The figure shows three views and two pictorial views of one solid part (mm, origin at its lowest corner). Answer the questions. A direction names the side the tool comes from. Give positions to 0.01 mm unless a question says otherwise; leave off trailing zeros. Order: outer loops, then holes, each group sorted by start corner. A loop starts at its lowest first (then second) coordinate and runs counter-clockwise, first axis right, second up. Notation, with made-up numbers: (30, 12.5) - (58, 12.5) arc R9 cw to (58, 26.5) - close; hole circle Ø7 at (84, -27). An arc over 180 degrees is marked (long way). Write item = value, one per line.
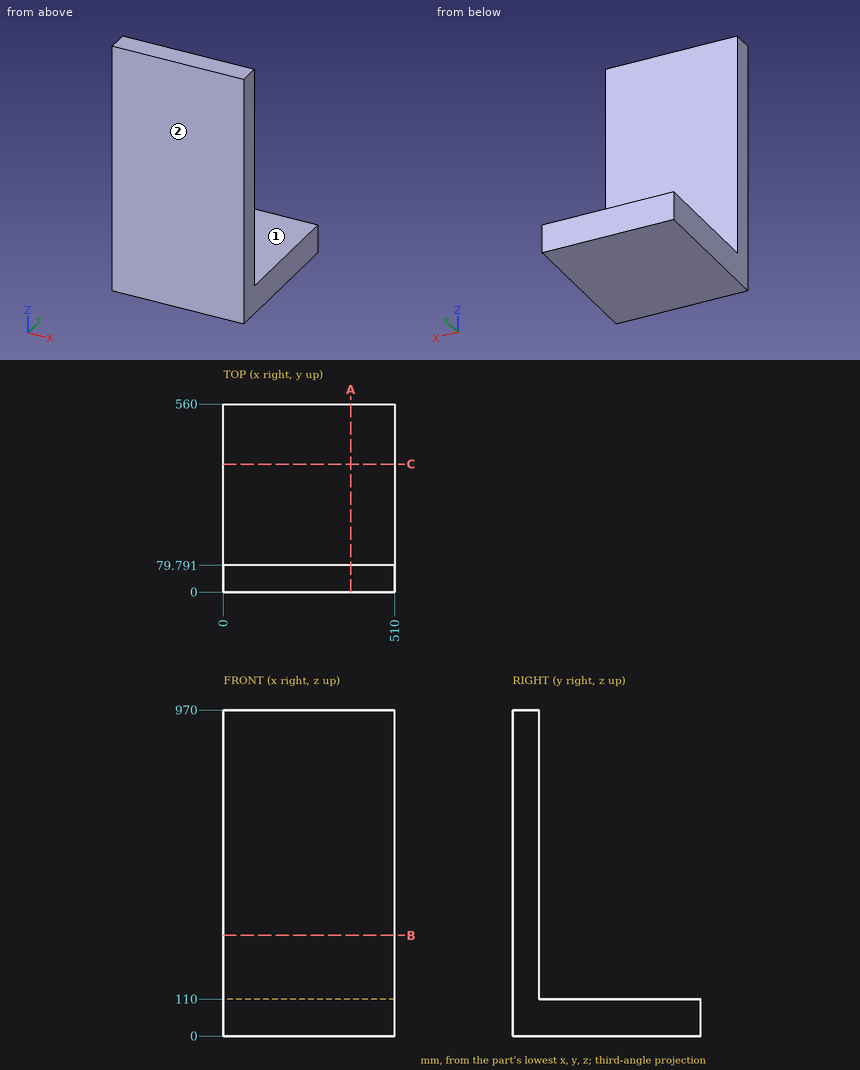
1. Flat-ended cylindrical pins translate along their axes: pin 1 (5 mm diameter, centred on x = 380, z = 136.5, fed in from +Y); pin 2 (6 mm diameter, centred on x = 432, y = 120, fed in from +Z). Find the tip coordinate at first contact, or state that the pin passes through.
Recorded:
pin_1 = 79.79
pin_2 = 110
2. Section C-C (y = 381) is taken. Determine the outline of the cut face in (x, z).
Recorded:
outline = (0, 0) - (510, 0) - (510, 110) - (0, 110) - close
3. Section A-A (x = 380) is taken. Determine the outline of the cut face in (y, z).
Recorded:
outline = (0, 0) - (560, 0) - (560, 110) - (79.79, 110) - (79.79, 970) - (0, 970) - close
4. Section B-B (z = 299.5) is taken. Determine the outline of the cut face in (x, y).
Recorded:
outline = (0, 0) - (510, 0) - (510, 79.79) - (0, 79.79) - close
5. For the marked faces 1 and 2, determine the directions among +Z, -Z, +X, -X, +Y, -Y from which every point of the face is accessible in a straight line to the end or side of a thin tool.
Recorded:
face_1 = +Z, +X, -X, +Y
face_2 = +Z, -Z, +X, -X, -Y
6. Straight lines are drawn through the part: L1, parallel to Z at x = 72, y = 468; L2, parallel to Y at x = 78.5, z = 394.5. For each, find the intervals that lie inside material, in ascending order. Write a range as [from, to].
Recorded:
L1 = [0, 110]
L2 = [0, 79.79]
